from build123d import *

# Parameters (mm, degrees)
F1_DEPTH = 4
F2_R     = 3.25
F3_DEPTH = 4.001


with BuildPart() as f1:
    # F0 (on Front) → F1 (new body)
    with BuildSketch(Plane.XZ):
        with BuildLine():
            Line((25, 35), (-25, 35))
            ThreePointArc((-25, 35), (-60, 0), (-25, -35))
            Line((-25, -35), (25, -35))
            ThreePointArc((25, -35), (60, 0), (25, 35))
        make_face()
    extrude(amount=F1_DEPTH)

    # F2 (on Front) → F3 (cut, through all)
    with BuildSketch(Plane.XZ):
        with Locations((-21, 31)):
            Circle(F2_R)
        with Locations((21, -31)):
            Circle(F2_R)
        with Locations((53.5, 0)):
            Circle(F2_R)
        with Locations((-53.5, 0)):
            Circle(F2_R)
    extrude(amount=F3_DEPTH, mode=Mode.SUBTRACT)


solid = f1.part
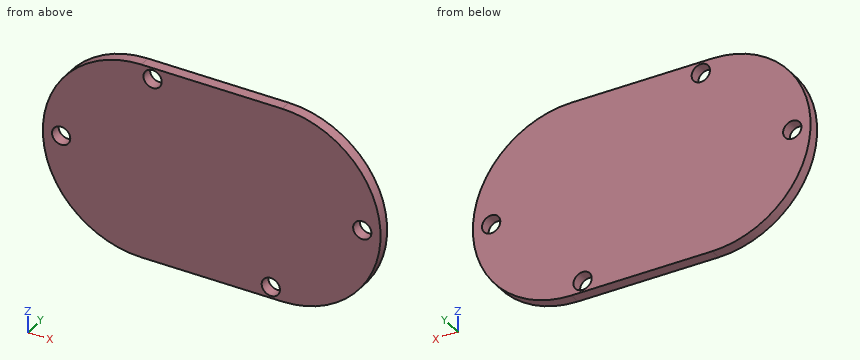
Design review of the part built by this model. Coordinates are the model's own, in mm. Round coordinates to 2 decimals unless told otherwise and drop trailing zeros. Write each loop counter-clockwise with the first axis right and the second up, starting at its lowest first coordinate (ties: lowest second). Pieces come first, ordered by that corner, then holes. Notation, with made-up numbers: (81, -25.75) - (111, -25.75) arc R4 cw to (111, -19.75) - close; hole circle Ø11 at (19.5, 21). An arc over 180 degrees is marked (long way). Use a Markdown table: item, result. Add a question column.
1. We need section D-D (z = 31). State the section outline as (x, y) points.
2. Clearance check with a flat-ended pin moving along its axis: pin 1 (1.5 mm diameter, centred on y = -1.5, z = -26, fed in from +X). State where the tip first meets the part, or that it passes through.
3. We need section B-B (x = 21). State the section outline as (y, z) points, then the cut area to 3 significant figures.
4. We need section C-C (y = -2.65). State the section outline as (x, z) points.
5. We need section A-A (z = 0). State the section outline as (x, y) points.
6. Wall thickness on probe 1 along X at (y, z) = (-1.25, 0); probe 2 along Z at (x, y) = (21, -1); probe 3 along Z at (x, y) = (-53.5, -1.9): over which ranges is each line inside the solid? List them lowest first.
Output:
| question | item | result |
|---|---|---|
| 1 | outline | (-41.25, -4) - (-24.25, -4) - (-24.25, 0) - (-41.25, 0) - close; (-17.75, -4) - (41.25, -4) - (41.25, 0) - (-17.75, 0) - close |
| 2 | pin 1 | stops at x = 49.24 |
| 3 | outline | (-4, -35) - (0, -35) - (0, -34.25) - (-4, -34.25) - close; (-4, -27.75) - (0, -27.75) - (0, 35) - (-4, 35) - close |
| 3 | area | 254 mm2 |
| 4 | outline | (-25, -35) - (25, -35) arc R35 ccw to (25, 35) - (-25, 35) arc R35 ccw to start; hole circle Ø6.5 at (-53.5, 0); hole circle Ø6.5 at (-21, 31); hole circle Ø6.5 at (21, -31); hole circle Ø6.5 at (53.5, 0) |
| 5 | outline | (-60, -4) - (-56.75, -4) - (-56.75, 0) - (-60, 0) - close; (-50.25, -4) - (50.25, -4) - (50.25, 0) - (-50.25, 0) - close; (56.75, -4) - (60, -4) - (60, 0) - (56.75, 0) - close |
| 6 | probe 1 | x = -60 to -56.75, -50.25 to 50.25, 56.75 to 60 |
| 6 | probe 2 | z = -35 to -34.25, -27.75 to 35 |
| 6 | probe 3 | z = -20.32 to -3.25, 3.25 to 20.32 |
